Part model, mm, in its own coordinate system. A direction names the side the tool comes from. Coordinates: 2 decimals unless noted, no trailing zeros. Write each loop counter-clockwise with the first axis right and the second up, starting at its lowest first coordinate (ties: lowest second). Pieces come first, ordered by that corner, then holes. Notation, with made-up numbers: (66.25, 80.25) -> (123.25, 80.25) arc R8 cw to (123.25, 90.25) -> close; hole circle Ø8 at (-7, -35). An arc over 180 degrees is marked (long way). One line per question, with ' | ' between items. Start each with the question number.
Item 1: Two-plate mould, pull along Y, no slides. Class faces 1 (the flat face through (-256, -250, 26)), 2 (the flat face through (-256, -3, -50)), 3 (the cylindrical face through (-256.084, 6.014, 377.703)): pulls with the +Y half, pulls with the -Y half, needs draft (parallel to the pull), parting line crosses it, or undercut.
Item 2: 3-axis set-ups, long thin cutter, end or side, ignore diameter. For faces 4 (the flat face through (-256, 73, 452)), 5 (the cylindrical face through (-255.916, 134.297, 405.986)): which of +Z, -Z, +X, -X, +Y, -Y reach the whole face in a straight line?
Item 3: Pin check, flat tips, straight feed: pin 1 (5 mm diameter, centred on x = -260, z = 204.5, fed in from -Y); pin 2 (1.5 mm diameter, centred on x = -257, z = 327, fed in from -Y). Stop position of each tip, or through.
Item 4: Saw through at C-C (z = 385). List the corners of the cut face in (x, y) (3 decimals).
Item 5: Saw through at D-D (y = -150.5). List the corners of the cut face in (x, z), and give its area (3 significant figures).
Item 6: Probe probe 1 along Z at (x, y) = (-261, 32); probe 2 along Y at (x, z) = (-255.5, 382); probe 3 along Z at (x, y) = (-254.5, 136). List the from-to ranges inside material, lowest first. Write a range as [from, to].
Item 7: Saw through at A-A (y = 100). List the corners of the cut face in (x, z), and give its area (3 significant figures).
from build123d import *

# Parameters (mm, degrees)
F0_W      = 500
F0_H      = 500
F1_DEPTH  = 12
F2_W      = 500
F2_H      = 50
F3_DEPTH  = 6
F6_DEPTH  = 6
F14_DEPTH = 6
F15_R     = 19.99999
F19_DEPTH = 6
F22_DEPTH = 12
F25_DEPTH = 6
F27_W     = 12
F27_H     = 320
F28_DEPTH = 44
F31_W     = 196
F31_H     = 12
F32_DEPTH = 44
F37_DEPTH = 3
F43_DEPTH = 12


# Not quite as in the source:
# - a fillet or chamfer is up to 0.001 mm smaller than in the source, because OpenCascade refuses the exact size


with BuildPart() as f1:
    # F0 (on Top) → F1 (new body)
    with BuildSketch(Plane.XY):
        Rectangle(F0_W, F0_H)
    extrude(amount=F1_DEPTH)


with BuildPart() as f3:
    # F2 (on Right) → F3 (new body, symmetric)
    with BuildSketch(Plane.YZ):
        Rectangle(F2_W, F2_H)
    extrude(amount=F3_DEPTH, both=True)


with BuildPart() as f3_1:
    # F4: moved
    add(f3.part.moved(Location((0, 0, -25))))


with BuildPart() as f6:
    # F5 (on Front) → F6 (new body, symmetric)
    with BuildSketch(Plane.XZ):
        Polygon((-250, -25), (250, -25), (250, 25), (6, 25), (6, 0), (-6, 0), (-6, 25), (-250, 25), align=None)
    extrude(amount=F6_DEPTH, both=True)


with BuildPart() as f6_1:
    # F7: moved
    add(f6.part.moved(Location((0, 80, -25))))


with BuildPart() as f8_1:
    # F8: copy of F6
    add(f6_1.part)


with BuildPart() as f3_2:
    add(f3_1.part)

    # F10: cut F6
    add(f6_1.part, mode=Mode.SUBTRACT)


with BuildPart() as f11_1:
    # F11: copy of F6
    add(f6_1.part.moved(Location((0, 164, 0))))


with BuildPart() as f3_3:
    add(f3_2.part)

    # F12: cut F11_1
    add(f11_1.part, mode=Mode.SUBTRACT)


with BuildPart() as f14:
    # F13 (on Right) → F14 (new body, symmetric)
    with BuildSketch(Plane.YZ):
        Polygon((250, -50), (250, 0), (250, 452), (70, 452), (-110, 452), (-250, 100), (-250, -50), align=None)
        Polygon((0, 412), (70, 412), (140, 412), (140, 372), (0, 372), align=None, mode=Mode.SUBTRACT)
    extrude(amount=F14_DEPTH, both=True)

    # F15 (radius 20 in the source; OpenCascade refuses exactly that, so slightly less here)
    f15_edges = [f14.edges().sort_by_distance(p)[0] for p in [
        (0, 140, 372),
        (0, 140, 412),
        (0, 0, 412),
        (0, 0, 372),
    ]]
    fillet(f15_edges, radius=F15_R)


with BuildPart() as f14_1:
    # F16: moved
    add(f14.part.moved(Location((-256, 0, 0))))


with BuildPart() as f17_1:
    # F17: copy of F14
    add(f14_1.part.moved(Location((512, 0, 0))))


with BuildPart() as f19:
    # F18 (on Front) → F19 (new body, symmetric)
    with BuildSketch(Plane.XZ):
        Polygon((-262, 452), (-262, 0), (-262, -50), (262, -50), (262, 452), align=None)
    extrude(amount=F19_DEPTH, both=True)


with BuildPart() as f19_1:
    # F20: moved
    add(f19.part.moved(Location((0, 256, 0))))


with BuildPart() as f22:
    # F21 (on face) → F22 (new body)
    with BuildSketch(Plane.XY.offset(12)):
        Polygon((262, 262), (0, 262), (-262, 262), (-262, -110), (262, -110), align=None)
    extrude(amount=F22_DEPTH)


with BuildPart() as f22_1:
    # F23: moved
    add(f22.part.moved(Location((0, 0, 440))))


with BuildPart() as f25:
    # F24 (on Front) → F25 (new body, symmetric)
    with BuildSketch(Plane.XZ):
        Polygon((-250, 12), (0, 12), (250, 12), (250, 100), (-250, 100), align=None)
    extrude(amount=F25_DEPTH, both=True)


with BuildPart() as f25_1:
    # F26: moved
    add(f25.part.moved(Location((0, -244, 0))))


with BuildPart() as f28:
    # F27 (on Top) → F28 (new body)
    with BuildSketch(Plane.XY):
        with Locations((-24, -90)):
            Rectangle(F27_W, F27_H)
    extrude(amount=F28_DEPTH)


with BuildPart() as f28_1:
    # F29: moved
    add(f28.part.moved(Location((0, 0, -48))))


with BuildPart() as f30_1:
    # F30: copy of F28
    add(f28_1.part.moved(Location((-208, 0, 0))))


with BuildPart() as f32:
    # F31 (on Top) → F32 (new body)
    with BuildSketch(Plane.XY):
        with Locations((-128, -244)):
            Rectangle(F31_W, F31_H)
    extrude(amount=-F32_DEPTH)


with BuildPart() as f32_1:
    # F33: moved
    add(f32.part.moved(Location((0, 0, -4))))


with BuildPart() as f34_1:
    # F34: copy of F32
    add(f32_1.part.moved(Location((0, 308, 0))))


with BuildPart() as f35_1:
    # F35: copy of F32
    add(f32_1.part.moved(Location((256, 0, 0))))


with BuildPart() as f35_2:
    # F35: copy of F30_1
    add(f30_1.part.moved(Location((256, 0, 0))))


with BuildPart() as f35_3:
    # F35: copy of F28
    add(f28_1.part.moved(Location((256, 0, 0))))


with BuildPart() as f35_4:
    # F35: copy of F34_1
    add(f34_1.part.moved(Location((256, 0, 0))))


with BuildPart() as f37:
    # F36 (on Top) → F37 (new body)
    with BuildSketch(Plane.XY):
        Polygon((-24, -244), (-24, 0), (-24, 64), (-232, 64), (-232, -244), align=None)
    extrude(amount=F37_DEPTH)


with BuildPart() as f37_1:
    # F38: moved
    add(f37.part.moved(Location((0, 0, -44))))


with BuildPart() as f39_1:
    # F39: copy of F37
    add(f37_1.part.moved(Location((256, 0, 0))))


with BuildPart() as f30_1_1:
    add(f30_1.part)

    # F40: cut F37
    add(f37_1.part, mode=Mode.SUBTRACT)


with BuildPart() as f32_2:
    add(f32_1.part)

    # F40: cut F37
    add(f37_1.part, mode=Mode.SUBTRACT)


with BuildPart() as f28_2:
    add(f28_1.part)

    # F40: cut F37
    add(f37_1.part, mode=Mode.SUBTRACT)


with BuildPart() as f34_1_1:
    add(f34_1.part)

    # F40: cut F37
    add(f37_1.part, mode=Mode.SUBTRACT)


with BuildPart() as f35_1_1:
    add(f35_1.part)

    # F41: cut F39_1
    add(f39_1.part, mode=Mode.SUBTRACT)


with BuildPart() as f35_3_1:
    add(f35_3.part)

    # F41: cut F39_1
    add(f39_1.part, mode=Mode.SUBTRACT)


with BuildPart() as f35_4_1:
    add(f35_4.part)

    # F41: cut F39_1
    add(f39_1.part, mode=Mode.SUBTRACT)


with BuildPart() as f35_2_1:
    add(f35_2.part)

    # F41: cut F39_1
    add(f39_1.part, mode=Mode.SUBTRACT)


with BuildPart() as f43:
    # F42 (on Front) → F43 (new body)
    with BuildSketch(Plane.XZ):
        Polygon((0, 12), (0, 0), (0, -50), (262, -50), (262, 12), align=None)
    extrude(amount=F43_DEPTH)


with BuildPart() as f43_1:
    # F44: moved
    add(f43.part.moved(Location((0, -250, 0))))


with BuildPart() as f45_1:
    # F45: copy of F43
    add(f43_1.part.moved(Location((-262, 0, 0))))


solid = f14_1.part
From the geometry:
1) face 1: pulls with the -Y half | face 2: needs draft | face 3: undercut
2) face 4: +Z, +X, -X, +Y, -Y | face 5: +X, -X
3) pin 1: y = -209.43 | pin 2: y = -160.01
4) outline: (-262, -136.648) -> (-250, -136.648) -> (-250, 1.265) -> (-262, 1.265) -> close; (-262, 138.735) -> (-250, 138.735) -> (-250, 250) -> (-262, 250) -> close
5) outline: (-262, -50) -> (-250, -50) -> (-250, 350.17) -> (-262, 350.17) -> close | area: 4,800 mm2
6) probe 1: [-50, 372], [412, 452] | probe 2: [-137.84, 2.68], [137.32, 250] | probe 3: [-50, 380], [404, 452]
7) outline: (-262, -50) -> (-250, -50) -> (-250, 372) -> (-262, 372) -> close; (-262, 412) -> (-250, 412) -> (-250, 452) -> (-262, 452) -> close | area: 5,540 mm2
